from build123d import *

# Parameters (mm, degrees)
F0_W     = 2
F0_H     = 40
F1_DEPTH = 45
F2_R     = 5
F3_R     = 5


with BuildPart() as f1:
    # F0 (on Right) → F1 (new body, symmetric)
    with BuildSketch(Plane.YZ):
        with Locations((0, 20.7)):
            Rectangle(F0_W, F0_H)
        Polygon((30, -0.7), (30, 0.7), (1, 0.7), (-1, 0.7), (-30, 0.7), (-30, -0.7), align=None)
    extrude(amount=F1_DEPTH, both=True)

    # F2
    f2_edges = [f1.edges().sort_by_distance(p)[0] for p in [
        (0, -1, 0.7),
        (0, 1, 0.7),
    ]]
    fillet(f2_edges, radius=F2_R)

    # F3
    f3_edges = [f1.edges().sort_by_distance(p)[0] for p in [
        (-45, -30, 0),
        (-45, 30, 0),
        (45, 30, 0),
        (45, -30, 0),
        (-45, 0, 40.7),
        (45, 0, 40.7),
    ]]
    fillet(f3_edges, radius=F3_R)


solid = f1.part
Geometry: final body of the model. Coordinates: model frame, mm. A direction names the side the tool comes from. Round coordinates to 2 decimals unless told otherwise and drop trailing zeros. Loops run counter-clockwise (first coordinate to the right, second up) from the corner with the lowest first, then second, coordinate; pieces in that order, holes last.
Q1. Material intervals for L1, parallel to Z at x = 35.5, y = -15.5; L2, parallel to Y at x = 9.5, z = 9; L3, parallel to Z at x = 33, y = 4, sorted ascending.
Q2. Access query for faces 1 (the cylindrical face through (-43.57, 0.01, 39.2)), 2 (the flat face through (1, -1, 23)), 3 (the flat face through (1, 18, 0.7)). Directions: +Z, -Z, +X, -X, +Y, -Y. A direction counts if a zero-diameter tool reaches every point of the face in a straight line with its end or side. Return the directions, or none.
Q3. Section B-B on y = 19.5. Return loops of the section in (x, z), plus the area to 3 significant figures.
Q4. Section C-C on z = 8. Return loops of the section in (x, y), plus the area to 3 significant figures.
Q5. Section A-A on x = -9. Return loops of the section in (y, z).
Q6. Pin query (flat end, axial travel): P1, Ø1.5, axis at x = -2, z = 6.5, coming from the -Y side; P2, Ø6, axis at x = -16, z = 5.5, coming from the -Y side; P3, Ø12, axis at y = -11.5, z = 15, coming from the +X side; P4, Ø12, axis at x = 7, y = -19.5, coming from the +Z side. Return the tip coordinate at first contact, or that it passes through.
Evaluation:
1. L1: z = -0.7 to 0.7
1. L2: y = -1 to 1
1. L3: z = -0.7 to 1.12
2. face 1: +Z, -X, +Y, -Y
2. face 2: +Z, +X, -X, -Y
2. face 3: +Z, +X, -X, +Y
3. outline: (-45, -0.7) - (45, -0.7) - (45, 0.7) - (-45, 0.7) - close
3. area: 126 mm2
4. outline: (-45, -1) - (45, -1) - (45, 1) - (-45, 1) - close
4. area: 180 mm2
5. outline: (-30, -0.7) - (30, -0.7) - (30, 0.7) - (6, 0.7) arc R5 cw to (1, 5.7) - (1, 40.7) - (-1, 40.7) - (-1, 5.7) arc R5 cw to (-6, 0.7) - (-30, 0.7) - close
6. P1: stops at y = -1
6. P2: stops at y = -2.16
6. P3: passes through
6. P4: stops at z = 0.7
